Design review of the part built by this model. Coordinates are the model's own, in mm. Face numbers are marked on the shaded views. A direction names the side the tool comes from. Coordinates: 2 decimals unless noted, no trailing zeros. Loops run counter-clockwise (first coordinate to the right, second up) from the corner with the lowest first, then second, coordinate; pieces in that order, holes last. Notation, with made-up numbers: M -18,59.25 L 21,59.25 A25 ccw 21,75.25 Z; hole C 11.25,-36 d7. An arc over 180 degrees is marked long. Answer as CSV lines item,"result". Start each with the question number.
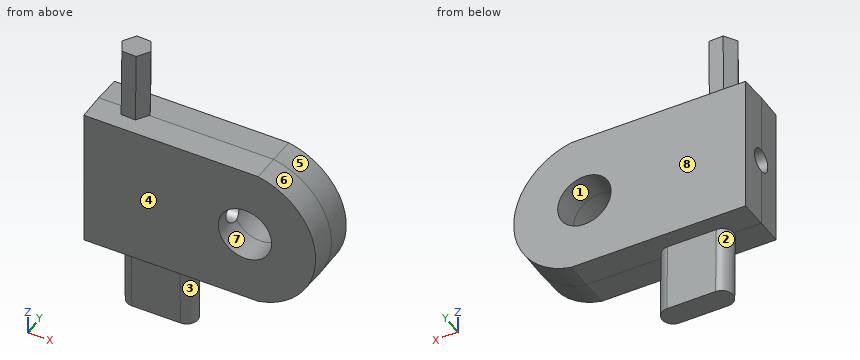
from build123d import *

# Parameters (mm, degrees)
SKETCH1_R                     = 15
BOSS_EXTRUDE1_DEPTH           = 15.54000612
BOSS_EXTRUDE1_DRAFT           = 1
BOSS_EXTRUDE1_OTHER_WAY_DEPTH = 15.54000612
BOSS_EXTRUDE1_OTHER_WAY_DRAFT = -1
SKETCH4_R                     = 6.744646555
CUT_EXTRUDE3_DEPTH            = 93.319796338
BOSS_EXTRUDE4_DEPTH           = 40
BOSS_EXTRUDE5_DEPTH           = 40


with BuildPart() as part:
    # Sketch1 → Boss-Extrude1 (with draft: the straight prism first)
    with BuildSketch(Plane(origin=(0, 0, 0), x_dir=(1, 0, 0), z_dir=(0, 1, 0))):
        with BuildLine():
            Line((-20.823660635, 37.109004739), (-20.823660635, -42.890995261))
            Line((-20.823660635, -42.890995261), (79.176339365, -42.890995261))
            ThreePointArc((79.176339365, -42.890995261), (112.281888642, -2.890995261), (79.176339365, 37.109004739))
            Line((79.176339365, 37.109004739), (-20.823660635, 37.109004739))
        make_face()
        with Locations((71.563981043, -2.890995261)):
            Circle(SKETCH1_R, mode=Mode.SUBTRACT)
    extrude(amount=BOSS_EXTRUDE1_DEPTH)
    # Boss-Extrude1: the draft: its side faces are tilted about the plane it starts from
    boss_extrude1_sides = [part.faces().sort_by_distance(p)[0] for p in [
        (29.176339365, 7.77000306, -37.109004739),
        (-20.823660635, 7.77000306, 2.890995261),
        (29.176339365, 7.77000306, 42.890995261),
        (112.281888642, 7.77000306, 2.890995261),
        (56.563981043, 7.77000306, 2.890995261),
    ]]
    draft(boss_extrude1_sides, Plane(origin=(0, 0, 0), x_dir=(1, 0, 0), z_dir=(0, 1, 0)), BOSS_EXTRUDE1_DRAFT)


with BuildPart() as boss_extrude1_other_way_tool:
    # Sketch1 → Boss-Extrude1 other way (with draft: the straight prism first)
    with BuildSketch(Plane(origin=(0, 0, 0), x_dir=(1, 0, 0), z_dir=(0, 1, 0))):
        with BuildLine():
            Line((-20.823660635, 37.109004739), (-20.823660635, -42.890995261))
            Line((-20.823660635, -42.890995261), (79.176339365, -42.890995261))
            ThreePointArc((79.176339365, -42.890995261), (112.281888642, -2.890995261), (79.176339365, 37.109004739))
            Line((79.176339365, 37.109004739), (-20.823660635, 37.109004739))
        make_face()
        with Locations((71.563981043, -2.890995261)):
            Circle(SKETCH1_R, mode=Mode.SUBTRACT)
    extrude(amount=-BOSS_EXTRUDE1_OTHER_WAY_DEPTH)
    # Boss-Extrude1 other way: the draft: its side faces are tilted about the plane it starts from
    boss_extrude1_other_way_sides = [boss_extrude1_other_way_tool.faces().sort_by_distance(p)[0] for p in [
        (29.176339365, -7.77000306, -37.109004739),
        (-20.823660635, -7.77000306, 2.890995261),
        (29.176339365, -7.77000306, 42.890995261),
        (112.281888642, -7.77000306, 2.890995261),
        (56.563981043, -7.77000306, 2.890995261),
    ]]
    draft(boss_extrude1_other_way_sides, Plane(origin=(0, 0, 0), x_dir=(1, 0, 0), z_dir=(0, 1, 0)), BOSS_EXTRUDE1_OTHER_WAY_DRAFT)


with BuildPart() as part_1:
    add(part.part)

    # Boss-Extrude1 other way: add boss_extrude1_other_way_tool
    add(boss_extrude1_other_way_tool.part)

    # Sketch4 → Cut-Extrude3 (cut)
    with BuildSketch(Plane(origin=(-20.817318029, 0.363367638, 0), x_dir=(0, 0, 1), z_dir=(-0.9998476951563913, 0.01745240643728355, 0))):
        with Locations((2.890995261, -0.363422989)):
            Circle(SKETCH4_R)
    extrude(amount=-CUT_EXTRUDE3_DEPTH, mode=Mode.SUBTRACT)

    # Sketch5 → Boss-Extrude4 (add)
    with BuildSketch(Plane(origin=(0, 0.647542794, -37.097701838), x_dir=(-1, 0, 0), z_dir=(0, 0.01745240643728355, -0.9998476951563913))):
        with BuildLine():
            Line((-29.176339365, 5.74353059), (-1.322649043, 5.74353059))
            ThreePointArc((-1.322649043, 5.74353059), (5.06852298, -0.647641433), (-1.322649043, -7.038813456))
            Line((-1.322649043, -7.038813456), (-29.176339365, -7.038813456))
            ThreePointArc((-29.176339365, -7.038813456), (-35.567511388, -0.647641433), (-29.176339365, 5.74353059))
        make_face()
    extrude(amount=BOSS_EXTRUDE4_DEPTH)

    # Sketch6 → Boss-Extrude5 (add)
    with BuildSketch(Plane(origin=(0, 0.748437074, 42.877931243), x_dir=(1, 0, 0), z_dir=(0, 0.017452406437283557, 0.9998476951563913))):
        Polygon((3.92205187, -7.356373004), (8.331831836, -0.281589948), (4.409779966, 7.074783056), (-3.92205187, 7.356373004), (-8.331831836, 0.281589948), (-4.409779966, -7.074783056), align=None)
    extrude(amount=BOSS_EXTRUDE5_DEPTH)


solid = part_1.part
Item 1: For pin 1 (10 mm diameter, centred on y = 2, z = 2.5, fed in from -X); pin 2 (2 mm diameter, centred on x = 24.5, y = 2, fed in from +Z); pin 3 (8 mm diameter, centred on y = 9, z = -60.5, fed in from -X), all flat-tipped, find the tip position at first contact; note any pin that passes through.
Item 2: Add section A-A (y = 13). Give the boundary of the cut face in (x, z).
Item 3: For the marked faces 1, 2, 3, 4 and 5, list the 3-axis set-ups (+Z, -Z, +X, -X, +Y, -Y) from which the entire face can be reached by the end or side of a thin tool; tool diameter is ignored.
Item 4: Mouldability with a two-part tool opening along X and no side actions: class the marked faces 6, 7 and 8 as released by +X, released by -X, zero draft, split by the parting line, or undercut.
Item 5: Add section C-C (z = 1). Give the number of separate pieces and of enclosed holes in the cut face, plus the area to 3 significant figures.
Item 6: For line 1 along Z through (x, y) = (57, -2); line 2 along Z through (x, y) = (37, -5.5) (3 decimals); line 3 along Z through (x, y) = (27, -8), list the stretches that pass through material, from the lowest coordinate up. Write a range as from..to.
Item 7: Add section B-B (z = 59.5). Give the boundary of the cut face in (x, y).
Response:
1,pin 1,"x = -20.73"
1,pin 2,"z = 42.87"
1,pin 3,"x = -3.12"
2,outline,"M -20.6,-36.88 L 79.15,-36.88 A40.49 ccw 79.15,42.66 L -20.6,42.66 Z; hole C 71.56,2.89 d30.45"
3,face 1,"+Y"
3,face 2,"-X"
3,face 3,"+X"
3,face 4,"+Z, -Z, +X, -X, -Y"
3,face 5,"+X, +Y"
4,face 6,"released by +X"
4,face 7,"undercut"
4,face 8,"zero draft"
5,separate pieces,"3"
5,enclosed holes,"0"
5,area,"2,190 mm²"
6,line 1,"-37.07..-3.82, 9.61..42.86"
6,line 2,"-37.013..-2.142, 7.924..42.795"
6,line 3,"-36.97..42.75"
7,outline,"M -8.33,1.32 L -4.41,-6.04 L 3.92,-6.32 L 8.33,0.76 L 4.41,8.11 L -3.92,8.4 Z"
